```python
from build123d import *

# Parameters (mm, degrees)
ZAOKR_GLENIE1_R                  = 10
SZKIC2_R                         = 50.8
SZKIC2_R_2                       = 44.45
DODANIE_WYCI_GNI_CIE1_DEPTH      = 10
SZKIC3_R                         = 5.35
WYTNIJ_WYCI_GNI_CIE1_DEPTH       = 19.4
SFAZOWANIE1_SIZE                 = 1
SZYK_KO_OWY1_COUNT               = 12
SFAZOWANIE1_OF_SZYK_KO_OWY1_SIZE = 1


with BuildPart() as part:
    # Szkic1 → Obrót1 (revolve)
    with BuildSketch(Plane.XY, mode=Mode.PRIVATE) as obr_t1_sk:
        Polygon((0, 48.25), (40, 48.25), (40, 57.15), (23, 72.5), (0, 72.5), align=None)
    revolve(obr_t1_sk.sketch.rotate(Axis((0, 0, 0), (1, 0, 0)), 90), axis=Axis((0, 0, 0), (1, 0, 0)))

    # Zaokrąglenie1
    zaokr_glenie1_edges = [part.edges().sort_by_distance(p)[0] for p in [
        (23, 0, -72.5),
    ]]
    fillet(zaokr_glenie1_edges, radius=ZAOKR_GLENIE1_R)

    # Szkic2 → Dodanie-wyciągnięcie1 (add)
    with BuildSketch(Plane(origin=(40, 0, 0), x_dir=(0, 0, -1), z_dir=(1, 0, 0))):
        with Locations(Location((0, 0, 0), (0, 0, 180))):
            Circle(SZKIC2_R)
        Circle(SZKIC2_R_2, mode=Mode.SUBTRACT)
    extrude(amount=DODANIE_WYCI_GNI_CIE1_DEPTH)

    # Szkic3 → Wytnij-wyciągnięcie1 (cut)
    with BuildSketch(Plane.ZY):
        with Locations((0, 62.5)):
            Circle(SZKIC3_R)
    wytnij_wyci_gni_cie1 = extrude(amount=-WYTNIJ_WYCI_GNI_CIE1_DEPTH, mode=Mode.SUBTRACT)

    # Sfazowanie1
    sfazowanie1_edges = [part.edges().sort_by_distance(p)[0] for p in [
        (0, 62.5, -5.35),
    ]]
    chamfer(sfazowanie1_edges, length=SFAZOWANIE1_SIZE)

    # Szyk kołowy1: Wytnij-wyciągnięcie1 ×12 about axis
    szyk_ko_owy1_axis = Axis((0, 0, 0), (1, 0, 0))
    for i in range(1, SZYK_KO_OWY1_COUNT):
        add(wytnij_wyci_gni_cie1.rotate(szyk_ko_owy1_axis, i * 360 / SZYK_KO_OWY1_COUNT), mode=Mode.SUBTRACT)

    # Sfazowanie1 of Szyk kołowy1
    sfazowanie1_of_szyk_ko_owy1_edges = [part.edges().sort_by_distance(p)[0] for p in [
        (0, 56.801587737, 26.61676409),
        (0, 35.88323591, 51.451587737),
        (0, 5.35, 62.5),
        (0, -26.61676409, 56.801587737),
        (0, -51.451587737, 35.88323591),
        (0, -62.5, 5.35),
        (0, -56.801587737, -26.61676409),
        (0, -35.88323591, -51.451587737),
        (0, -5.35, -62.5),
        (0, 26.61676409, -56.801587737),
        (0, 51.451587737, -35.88323591),
    ]]
    chamfer(sfazowanie1_of_szyk_ko_owy1_edges, length=SFAZOWANIE1_OF_SZYK_KO_OWY1_SIZE)


solid = part.part
```
Source: CAD feature listing. Evaluate the final solid. Frame: model axes, mm. A direction names the side the tool comes from. Give positions to 0.01 mm unless a question says otherwise; leave off trailing zeros. Loops run counter-clockwise (first coordinate to the right, second up) from the corner with the lowest first, then second, coordinate; pieces in that order, holes last. Notation, with made-up numbers: M 22.25,20 L 37.25,20 A34 ccw 37.25,54 Z; hole C -6.75,89.25 d11. An arc over 180 degrees is marked long. Put each result on its own line as item: value.
Q1. Section B-B (x = 28.5). Return the cut outline in (y, z), and give its area (3 significant figures).
Response values:
outline: C 0,0 d135.07; hole C 0,0 d96.5
area: 7,010 mm²
Q2. Section C-C (x = 36). Return the cut outline in (y, z), and give its area (3 significant figures).
Response values:
outline: C 0,0 d121.52; hole C 0,0 d96.5
area: 4,280 mm²
Q3. Section A-A (x = 7). Count the separate pieces of the cut face and the enclosed holes in it, and give its area (3 significant figures).
Response values:
separate pieces: 1
enclosed holes: 13
area: 8,120 mm²
Q4. Pin query (flat end, axial travel): P1, Ø6.5, axis at y = 54.13, z = -31.25, coming from the -X side; P2, Ø6, axis at x = 28, y = -43.5, coming from the -Z side; P3, Ø1, axis at x = 11, z = -8.5, coming from the +Y side. Return the tip coordinate at first contact, or that it passes through.
Response values:
P1: stops at x = 19.4
P2: stops at z = -56.41
P3: stops at y = 72.06
Q5. Mould query, pull axis Y, two halves, no side actions, for faces 1 (the flat face through (19.4, -63, 0)), 2 (the conical face through (39.115, 51.411, 26.74)). Classes: released by +Y, released by -Y, zero draft, split by the parting line, or undercut.
Response values:
face 1: undercut
face 2: split by the parting line
Q6. Line query: probe 1 along Y at (x, z) = (8, 0); probe 2 along Z at (x, y) = (8, 31); probe 3 along Y at (x, z) = (3.5, -30). Output: solid intervals per line, ascending. Write a range as [from, to].
Response values:
probe 1: y = [-72.5, -67.85], [-57.15, -48.25], [48.25, 57.15], [67.85, 72.5]
probe 2: z = [-65.54, -59.47], [-48.78, -36.97], [36.97, 48.78], [59.47, 65.54]
probe 3: y = [-66, -59.33], [-48.92, -37.79], [37.79, 48.92], [59.33, 66]
Q7. Reachability of faces 3 (the flat face through (19.4, 0, -63)), 4 (the cylindrical face through (44.93, 13.352, -42.397)), 5 (the cylindrical face through (44.93, 45.07, 23.44)) from +Z, -Z, +X, -X, +Y, -Y: full face, straight path, thin tool, end or side. Return the list, or none.
Response values:
face 3: -X
face 4: +X, -X
face 5: +X
